```python
from build123d import *

# Parameters (mm, degrees)
SKETCH_1_W          = 100
SKETCH_1_H          = 100
EXTRUDE_1_DEPTH     = 40
SKETCH_36_W         = 94
SKETCH_36_H         = 94
CUT_EXTRUDE_2_DEPTH = 37
SKETCH_4_W          = 3
SKETCH_4_H          = 88
EXTRUDE_6_DEPTH     = 6
SKETCH_52_W         = 2.795133155
SKETCH_52_H         = 88
EXTRUDE_7_DEPTH     = 6
EXTRUDE_9_DEPTH     = 6
SKETCH_57_W         = 2.795133155
SKETCH_57_H         = 94
EXTRUDE_10_DEPTH    = 6


with BuildPart() as part:
    # 草图1 → 凸台-拉伸1 (new body)
    with BuildSketch(Plane(origin=(0, 0, 0), x_dir=(0, 0, -1), z_dir=(1, 0, 0))):
        with Locations((6.345177665, 10.178154254)):
            Rectangle(SKETCH_1_W, SKETCH_1_H)
    extrude(amount=EXTRUDE_1_DEPTH)

    # 草图36 → 切除-拉伸2 (cut)
    with BuildSketch(Plane(origin=(40, 0, 0), x_dir=(0, 0, -1), z_dir=(1, 0, 0))):
        with Locations((6.163819268, 10.178154254)):
            Rectangle(SKETCH_36_W, SKETCH_36_H)
    extrude(amount=-CUT_EXTRUDE_2_DEPTH, mode=Mode.SUBTRACT)

    # 草图4 → 凸台-拉伸6 (add)
    with BuildSketch(Plane.XY.offset(43.654822335)):
        with Locations((38.5, 10.178154254)):
            Rectangle(SKETCH_4_W, SKETCH_4_H)
    extrude(amount=-EXTRUDE_6_DEPTH)

    # 草图52 → 凸台-拉伸7 (add)
    with BuildSketch(Plane(origin=(0, 0, -56.345177665), x_dir=(-1, 0, 0), z_dir=(0, 0, -1))):
        with Locations((-38.602433422, 10.178154254)):
            Rectangle(SKETCH_52_W, SKETCH_52_H)
    extrude(amount=-EXTRUDE_7_DEPTH)

    # 草图56 → 凸台-拉伸9 (add)
    with BuildSketch(Plane.XZ.offset(39.821845746)):
        Polygon((40, 40.836180732), (37.204866845, 40.836180732), (37.204866845, -53.163819268), (40, -53.163819268), (40, -50.345177665), align=None)
    extrude(amount=-EXTRUDE_9_DEPTH)

    # 草图57 → 凸台-拉伸10 (add)
    with BuildSketch(Plane(origin=(0, 60.178154254, 0), x_dir=(1, 0, 0), z_dir=(0, 1, 0))):
        with Locations((38.602433422, 6.163819268)):
            Rectangle(SKETCH_57_W, SKETCH_57_H)
    extrude(amount=-EXTRUDE_10_DEPTH)


solid = part.part
```
Work out the finished part from the listing and answer in its coordinate system (mm). A direction names the side the tool comes from. Round coordinates to 2 decimals unless told otherwise and drop trailing zeros. Order: outer loops, then holes, each group sorted by start corner. A loop starts at its lowest first (then second) coordinate and runs counter-clockwise, first axis right, second up.
Q1. The mould has two halves that part along Z. Classify faces 1 (the flat face through (20, -36.822, -6)), 2 (the flat face through (20, 11, -56.345)), 3 (the flat face through (0, 11, -6)): pulls with the +Z half, pulls with the -Z half, needs draft (parallel to the pull), parting line crosses it, or undercut.
Solution:
face 1: undercut
face 2: pulls with the -Z half
face 3: needs draft
Q2. A cutting plane is placed at C-C, the plane x = 34.5. Determine the outline of the cut face in (y, z), then the cut area to 3 significant figures.
Solution:
outline: (-39.82, -56.35) - (60.18, -56.35) - (60.18, 43.65) - (-39.82, 43.65) - close; hole (-36.82, -53.16) - (57.18, -53.16) - (57.18, 40.84) - (-36.82, 40.84) - close
area: 1,160 mm2
Q3. A cutting plane is placed at A-A, the plane z = 20. Determine the outline of the cut face in (x, y).
Solution:
outline: (0, -39.82) - (40, -39.82) - (40, -33.82) - (37.2, -33.82) - (37.2, -36.82) - (3, -36.82) - (3, 57.18) - (37.2, 57.18) - (37.2, 54.18) - (40, 54.18) - (40, 60.18) - (0, 60.18) - close
Q4. A tool of negligible diameter and unlimited length cuts with its end or side. For faces 4 (the flat face through (20, 57.178, -6)), 5 (the flat face through (20, 11, 43.655)), 6 (the flat face through (39, -33.822, -6)), from which of +Z, -Z, +X, -X, +Y, -Y can it reach the whole face along a straight path? Write none if from no direction.
Solution:
face 4: none
face 5: +Z, +X, -X, +Y, -Y
face 6: +X
Q5. Find the intervals of material crossed by line 1 along Z through (x, y) = (8.5, 23); line 2 along Y through (x, z) = (12, -34); line 3 along X through (y, z) = (24.5, -43), in increasing order.
Solution:
line 1: z = -56.35 to -53.16, 40.84 to 43.65
line 2: y = -39.82 to -36.82, 57.18 to 60.18
line 3: x = 0 to 3
Q6. A cutting plane is placed at B-B, the plane y = 50.5. Determine the outline of the cut face in (x, z).
Solution:
outline: (0, -56.35) - (40, -56.35) - (40, -50.35) - (37.2, -50.35) - (37.2, -53.16) - (3, -53.16) - (3, 40.84) - (37, 40.84) - (37, 37.65) - (40, 37.65) - (40, 43.65) - (0, 43.65) - close
